from build123d import *

# Parameters (mm, degrees)
F0_R           = 5
F1_DEPTH       = 150
F3_DEPTH       = 15
F5_DEPTH       = 25
F6_R           = 2
F7_DEPTH       = 1.6
F7_DEPTH_BACK  = 6
F9_DEPTH       = 12
F10_R          = 2.25
F11_DEPTH      = 1.5
F11_DEPTH_BACK = 6.5
F13_DEPTH      = 2.501
F13_DEPTH_BACK = 7.501


with BuildPart() as f1:
    # F0 (on Top) → F1 (new body)
    with BuildSketch(Plane.XY):
        Circle(F0_R)
    extrude(amount=F1_DEPTH)

    # F2 (on face) → F3 (join)
    with BuildSketch(Plane(origin=(0, 0, 0), x_dir=(1, 0, 0), z_dir=(0, 0, -1))):
        with BuildLine():
            ThreePointArc((2.2, 4.4899888641), (1.1291713066, 4.8708286934), (0, 5))
            ThreePointArc((0, 5), (-1.1291713066, 4.8708286934), (-2.2, 4.4899888641))
            Line((-2.2, 4.4899888641), (-2.2, -4.4899888641))
            ThreePointArc((-2.2, -4.4899888641), (-1.1291713066, -4.8708286934), (0, -5))
            ThreePointArc((0, -5), (1.1291713066, -4.8708286934), (2.2, -4.4899888641))
            Line((2.2, -4.4899888641), (2.2, 4.4899888641))
        make_face()
    extrude(amount=F3_DEPTH)

    # F4 (on face) → F5 (cut)
    with BuildSketch(Plane.YZ.offset(2.2)):
        with BuildLine():
            Line((5, -15), (5, -10))
            ThreePointArc((5, -10), (4.8708286934, -11.1291713066), (4.4899888641, -12.2))
            Line((4.4899888641, -12.2), (4.4899888641, -15))
            Line((4.4899888641, -15), (5, -15))
        make_face()
        with BuildLine():
            Line((4.4899888641, -15), (4.4899888641, -12.2))
            ThreePointArc((4.4899888641, -12.2), (2.6457513111, -14.2426406871), (0, -15))
            Line((0, -15), (4.4899888641, -15))
        make_face()
        with BuildLine():
            Line((-4.4899888641, -15), (0, -15))
            ThreePointArc((0, -15), (-2.6457513111, -14.2426406871), (-4.4899888641, -12.2))
            Line((-4.4899888641, -12.2), (-4.4899888641, -15))
        make_face()
        with BuildLine():
            ThreePointArc((-4.4899888641, -12.2), (-4.8708286934, -11.1291713066), (-5, -10))
            Line((-5, -10), (-5, -15))
            Line((-5, -15), (-4.4899888641, -15))
            Line((-4.4899888641, -15), (-4.4899888641, -12.2))
        make_face()
    extrude(amount=-F5_DEPTH, mode=Mode.SUBTRACT)

    # F6 (on face) → F7 (join, two sides)
    with BuildSketch(Plane.YZ.offset(2.2)) as f7_sk:
        with Locations((0, -10)):
            Circle(F6_R)
    extrude(amount=F7_DEPTH)
    extrude(f7_sk.sketch, amount=-F7_DEPTH_BACK)

    # F8 (on face) → F9 (cut)
    with BuildSketch(Plane.XY.offset(150)):
        with BuildLine():
            ThreePointArc((2.5, 4.3301270189), (1.2940952255, 4.8296291314), (0, 5))
            ThreePointArc((0, 5), (-1.2940952255, 4.8296291314), (-2.5, 4.3301270189))
            Line((-2.5, 4.3301270189), (-2.5, -4.3301270189))
            ThreePointArc((-2.5, -4.3301270189), (-1.2940952255, -4.8296291314), (0, -5))
            ThreePointArc((0, -5), (1.2940952255, -4.8296291314), (2.5, -4.3301270189))
            Line((2.5, -4.3301270189), (2.5, 4.3301270189))
        make_face()
    extrude(amount=-F9_DEPTH, mode=Mode.SUBTRACT)

    # F10 (on face) → F11 (cut, two sides)
    with BuildSketch(Plane.YZ.offset(-2.5)) as f11_sk:
        with Locations((0, 145)):
            Circle(F10_R)
    extrude(amount=-F11_DEPTH, mode=Mode.SUBTRACT)
    extrude(f11_sk.sketch, amount=F11_DEPTH_BACK, mode=Mode.SUBTRACT)

    # F12 (on face) → F13 (cut, two sides)
    with BuildSketch(Plane.YZ.offset(-2.5)) as f13_sk:
        with BuildLine():
            ThreePointArc((0, 150), (2.5, 149.3301270189), (4.3301270189, 147.5))
            Line((4.3301270189, 147.5), (4.3301270189, 150))
            Line((4.3301270189, 150), (0, 150))
        make_face()
        with BuildLine():
            ThreePointArc((-4.3301270189, 147.5), (-2.5, 149.3301270189), (0, 150))
            Line((0, 150), (-4.3301270189, 150))
            Line((-4.3301270189, 150), (-4.3301270189, 147.5))
        make_face()
    extrude(amount=-F13_DEPTH, mode=Mode.SUBTRACT)
    extrude(f13_sk.sketch, amount=F13_DEPTH_BACK, mode=Mode.SUBTRACT)


solid = f1.part
Source: CAD feature listing. Evaluate the final solid. Frame: model axes, mm. A direction names the side the tool comes from. Round coordinates to 2 decimals unless told otherwise and drop trailing zeros. Loops run counter-clockwise (first coordinate to the right, second up) from the corner with the lowest first, then second, coordinate; pieces in that order, holes last. Notation, with made-up numbers: (-11.75, 86) - (22.25, 86) arc R21 ccw to (22.25, 98) - close; hole circle Ø10 at (55, -19.75). An arc over 180 degrees is marked (long way). Write item = value, one per line. Start each with the question number.
Item 1: Material intervals for line 1 (Z direction, x = -3.05, y = 0); line 2 (Z direction, x = -3, y = 1.5); line 3 (X direction, y = 2.25, z = 98), sorted ascending.
Item 2: Mould query, pull axis X, two halves, no side actions, for faces 4 (the face through (0, 0, 138)), 5 (the face through (3, 0, 0)), 6 (the face through (3.8, 0, -10)). Classes: released by +X, released by -X, zero draft, split by the parting line, or undercut.
Item 3: Reachability of faces 1 (the face through (-3.24, -0.488, 142.804)), 2 (the face through (2.5, -1, 142.8)), 3 (the face through (-3, 0, -8)) from +Z, -Z, +X, -X, +Y, -Y: full face, straight path, thin tool, end or side. Return the list, or none.
Item 4: Section query B-B on z = 109. Output: boundary loops of the cut face in (x, y), plus the area to 3 significant figures.
Item 5: First-contact query: pin 1 Ø1.3 at (y, z) = (1, 145.5) entering from +X; pin 2 Ø2 at (x, y) = (1, -2.5) entering from -Z; pin 3 Ø4.5 at (y, z) = (-0.5, -10.5) entering from -X; pin 4 Ø5 at (y, z) = (1, 36.5) entering from -X. Flat tips, straight axial feed; report the tip coordinate or a pass-through.
Item 6: Section query A-A on z = 145. Output: boundary loops of the cut face in (x, y).
Results list:
q1.line_1 = -12 to -8, 0 to 142.75, 147.25 to 150
q1.line_2 = -11.32 to -8.68, 0 to 143.32, 146.68 to 149.77
q1.line_3 = -4.47 to 4.47
q2.face_4 = undercut
q2.face_5 = zero draft
q2.face_6 = released by +X
q3.face_1 = none
q3.face_2 = +Z, +Y, -Y
q3.face_3 = -X
q4.outline = circle Ø10 at (0, 0)
q4.area = 78.5 mm²
q5.pin_1 = 4.99
q5.pin_2 = -14.77
q5.pin_3 = -3.8
q5.pin_4 = -5
q6.outline = (-4, -2.25) - (-4, 2.25) - (-2.5, 2.25) - (-2.5, 4.33) arc R5 ccw to (-2.5, -4.33) - (-2.5, -2.25) - close; (2.5, -4.33) arc R5 ccw to (2.5, 4.33) - (2.5, 2.25) - (4, 2.25) - (4, -2.25) - (2.5, -2.25) - close
